Could you check a few things on this drawing? It's one solid part, dimensions in mm from its lowest x, y, z. Give positions to 0.01 mm unless a question says otherwise; leave off trailing zeros. Order: outer loops, then holes, each group sorted by start corner. A loop starts at its lowest first (then second) coordinate and runs counter-clockwise, first axis right, second up. Notation, with made-up numbers: (-13, -5.5) -> (13, -5.5) arc R11 ccw to (13, 4.5) -> close; hole circle Ø6 at (75.25, 28.25). An arc over 180 degrees is marked (long way). Answer as CSV lines item,"result".
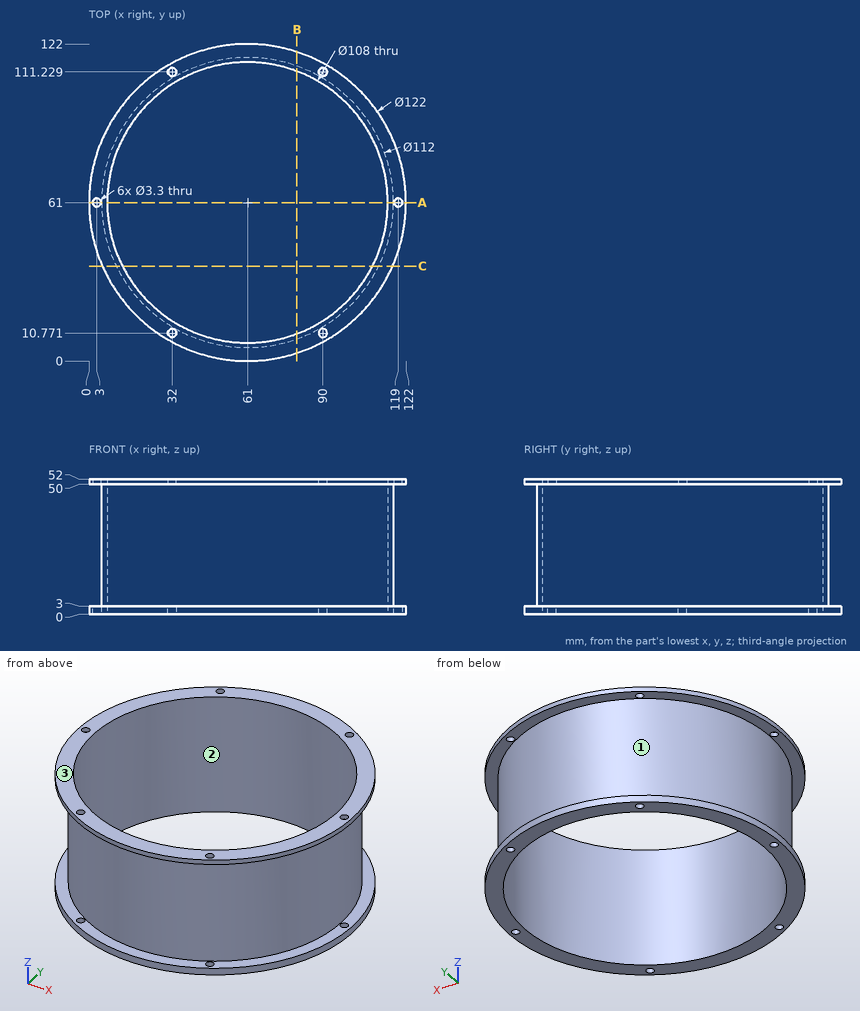
Item 1: We'd pull the mould along X, two halves only. Please class the marked faces 1, 2 and 3: released by +X, released by -X, zero draft, split by the parting line, or undercut.
Numbers:
face 1,"split by the parting line"
face 2,"undercut"
face 3,"zero draft"
Item 2: For pin 1 (5.5 mm diameter, centred on x = 32, y = 10.77, fed in from +Z); pin 2 (3 mm diameter, centred on x = 32, y = 111.23, fed in from +Z); pin 3 (3 mm diameter, centred on y = 101.5, z = 12, fed in from +X); pin 4 (1.5 mm diameter, centred on y = 75.5, z = 6, fed in from -X) (1 decimal), each with a flat end and sliding along its axis, tell me the tip position at first contact or that it passes through.
Numbers:
pin 1,"stops at z = 52"
pin 2,"passes through"
pin 3,"stops at x = 101.19"
pin 4,"stops at x = 6.7"
Item 3: Imagine slicing it at B-B, the plane x = 80. Please give me the cut outline in (y, z) (1 decimal).
Numbers:
outline,"(3, 0) -> (10.5, 0) -> (10.5, 52) -> (3, 52) -> (3, 50) -> (8.3, 50) -> (8.3, 3) -> (3, 3) -> close; (111.5, 0) -> (119, 0) -> (119, 3) -> (113.7, 3) -> (113.7, 50) -> (119, 50) -> (119, 52) -> (111.5, 52) -> close"
Item 4: Please list where these lines run through material, in increasing order: line 1 along Z through (x, y) = (40, 8); line 2 along Y through (x, z) = (40.5, 28.5); line 3 along Y through (x, z) = (54, 9.5) (1 decimal).
Numbers:
line 1,"z = 0 to 3, 50 to 52"
line 2,"y = 8.89 to 11.04, 110.96 to 113.11"
line 3,"y = 5.4 to 7.5, 114.5 to 116.6"
Item 5: Imagine slicing it at A-A, the plane y = 61. Give the number of separate pieces and of enclosed holes in the cut face, then the cut area to 3 significant figures.
Numbers:
separate pieces,"6"
enclosed holes,"0"
area,"225 mm²"
Item 6: Imagine slicing it at C-C, the plane y = 36.5. Please give me the cut outline in (x, z).
Numbers:
outline,"(5.14, 0) -> (12.88, 0) -> (12.88, 52) -> (5.14, 52) -> (5.14, 50) -> (10.64, 50) -> (10.64, 3) -> (5.14, 3) -> close; (109.12, 0) -> (116.86, 0) -> (116.86, 3) -> (111.36, 3) -> (111.36, 50) -> (116.86, 50) -> (116.86, 52) -> (109.12, 52) -> close"
